Geometry check sheet. Reference: the model listing, model coordinates, mm. Give positions to 0.01 mm unless a question says otherwise; leave off trailing zeros. Order: outer loops, then holes, each group sorted by start corner. A loop starts at its lowest first (then second) coordinate and runs counter-clockwise, first axis right, second up. Notation, with made-up numbers: M -12,25.25 L 44,25.25 A23 cw 44,46.25 Z; hole C 5.25,52.5 d9. An arc over 180 degrees is marked long. One line per question, with ' | ' between items. Start each with the question number.
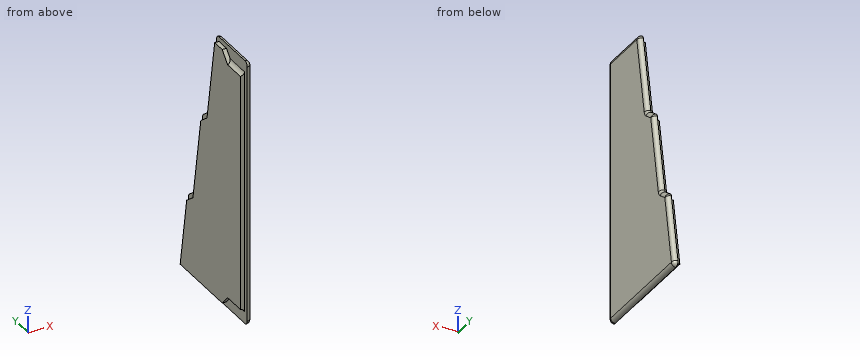
from build123d import *

# Parameters (mm, degrees)
BOSS_EXTRUDE1_DEPTH  = 3
FILLET1_R            = 3
BOSS_EXTRUDE2_DEPTH  = 3
CUT_EXTRUDE1_START   = -16.870694295
CUT_EXTRUDE1_DEPTH   = 17.870694295
CUT_EXTRUDE1_START_2 = 6.082684495
CUT_EXTRUDE1_2_DEPTH = 3.553569774
CUT_EXTRUDE1_START_3 = -94.677172909
CUT_EXTRUDE1_3_DEPTH = 3.677172909
CUT_EXTRUDE2_REACH   = 418.489


with BuildPart() as part:
    # Sketch1 → Boss-Extrude1 (new body)
    with BuildSketch(Plane.ZY.offset(376.423184311)):
        with BuildLine():
            Line((-33.382889261, -4.0880098), (-33.382889261, -11.0880098))
            ThreePointArc((-33.382889261, -11.0880098), (-32.504209605, -13.209330144), (-30.382889261, -14.0880098))
            Line((-30.382889261, -14.0880098), (147.429996243, -14.0880098))
            ThreePointArc((147.429996243, -14.0880098), (149.551316587, -13.209330144), (150.429996243, -11.0880098))
            Line((150.429996243, -11.0880098), (150.429996243, -4.0880098))
            Line((150.429996243, -4.0880098), (150.429996243, 23.394691306))
            ThreePointArc((150.429996243, 23.394691306), (149.728129572, 25.323054136), (147.950940776, 26.349114566))
            Line((147.950940776, 26.349114566), (92.565293245, 36.115098569))
            ThreePointArc((92.565293245, 36.115098569), (91.474338953, 36.539347491), (90.628781645, 37.348792519))
            Line((90.628781645, 37.348792519), (86.318516116, 43.504489644))
            ThreePointArc((86.318516116, 43.504489644), (85.472958808, 44.313934672), (84.382004516, 44.738183594))
            Line((84.382004516, 44.738183594), (27.741063701, 54.725509672))
            ThreePointArc((27.741063701, 54.725509672), (26.650109409, 55.149758594), (25.804552101, 55.959203622))
            Line((25.804552101, 55.959203622), (21.494286572, 62.114900747))
            ThreePointArc((21.494286572, 62.114900747), (20.648729264, 62.924345775), (19.557774972, 63.348594697))
            Line((19.557774972, 63.348594697), (-29.861944728, 72.062624659))
            ThreePointArc((-29.861944728, 72.062624659), (-32.31125209, 71.406334729), (-33.382889261, 69.1082014))
            Line((-33.382889261, 69.1082014), (-33.382889261, -4.0880098))
        make_face()
    extrude(amount=BOSS_EXTRUDE1_DEPTH)

    # Fillet1
    fillet1_edges = [part.edges().sort_by_distance(p)[0] for p in [
        (-379.423184311, 67.705609678, -5.152084878),
        (-379.423184311, 62.924345775, 20.648729264),
        (-379.423184311, 59.037052184, 23.649419336),
        (-379.423184311, 55.149758594, 26.650109409),
        (-379.423184311, 49.731846633, 56.061534109),
        (-379.423184311, 44.313934672, 85.472958808),
        (-379.423184311, 40.426641081, 88.473648881),
        (-379.423184311, 36.539347491, 91.474338953),
        (-379.423184311, 31.232106567, 120.258117011),
        (-379.423184311, 25.323054136, 149.728129572),
        (-379.423184311, 6.153340753, 150.429996243),
        (-379.423184311, -13.209330144, 149.551316587),
        (-379.423184311, -14.0880098, 58.523553491),
        (-379.423184311, -13.209330144, -32.504209605),
        (-379.423184311, 29.0100958, -33.382889261),
        (-379.423184311, 71.406334729, -32.31125209),
    ]]
    fillet(fillet1_edges, radius=FILLET1_R - 0.0001)  # a hair under: the kernel refuses the full size

    # Sketch2 → Boss-Extrude2 (add)
    with BuildSketch(Plane(origin=(-376.423184311, 0, 0), x_dir=(0, 0, -1), z_dir=(1, 0, 0))):
        Polygon((-147.129996243, 23.142961417), (-147.129996243, 13.236254269), (-143.529996243, 9.636254269), (-143.529996243, -4.0880098), (-143.529996243, -10.7880098), (26.482889261, -10.7880098), (26.482889261, -4.0880098), (26.482889261, 9.636254269), (30.082889261, 13.236254269), (30.082889261, 68.750675322), (-18.862359767, 60.120307341), (-24.598124131, 51.928786898), (-83.686589311, 41.509896238), (-89.422353675, 33.318375795), align=None)
    extrude(amount=BOSS_EXTRUDE2_DEPTH)

    # Cut-Extrude1: read off the stored shape, not the designer's step
    # Cut-Extrude1 outline → Cut-Extrude1 (cut)
    with BuildSketch(Plane.XZ.offset(10.7880098).offset(CUT_EXTRUDE1_START)):
        with BuildLine():
            Line((-376.423184311, 143.529996243), (-376.423184311, 142.329996243))
            ThreePointArc((-376.423184311, 142.329996243), (-375.230428102, 140.761580148), (-373.423184311, 139.97642647))
            Line((-373.423184311, 139.97642647), (-373.423184311, 143.529996243))
            Line((-373.423184311, 143.529996243), (-376.423184311, 143.529996243))
        make_face()
    extrude(amount=CUT_EXTRUDE1_DEPTH, mode=Mode.SUBTRACT)

    # Cut-Extrude1 2 outline → Cut-Extrude1 2 (cut)
    with BuildSketch(Plane(origin=(0, 0, 0), x_dir=(1, 0, 0), z_dir=(0, 1, 0)).offset(CUT_EXTRUDE1_START_2)):
        with BuildLine():
            ThreePointArc((-373.423184311, -139.97642647), (-375.230428102, -140.761580148), (-376.423184311, -142.329996243))
            Line((-376.423184311, -142.329996243), (-376.423184311, -143.529996243))
            Line((-376.423184311, -143.529996243), (-373.423184311, -143.529996243))
            Line((-373.423184311, -143.529996243), (-373.423184311, -139.97642647))
        make_face()
    extrude(amount=CUT_EXTRUDE1_2_DEPTH, mode=Mode.SUBTRACT)

    # Cut-Extrude1 3 outline → Cut-Extrude1 3 (add)
    with BuildSketch(Plane(origin=(0, 0, 0), x_dir=(1, 0, 0), z_dir=(0, 0.707106781186553, -0.707106781186542)).offset(CUT_EXTRUDE1_START_3)):
        with BuildLine():
            Line((-376.423184311, -106.607838111), (-376.423184311, -113.39606321))
            Line((-376.423184311, -113.39606321), (-373.423184311, -113.39606321))
            Line((-373.423184311, -113.39606321), (-373.423184311, -103.279387817))
            add(Edge.make_bspline(
                [(-373.423184311, -103.279387817), (-375.582623677, -103.754880716), (-376.423184311, -106.607838111)],
                knots=[0.154459598, 0.154459598, 0.154459598, 1.176005207, 1.176005207, 1.176005207], degree=2, weights=[1, 0.872366982, 1]))
        make_face()
    extrude(amount=CUT_EXTRUDE1_3_DEPTH)

    # Cut-Extrude2: up to this plane
    cut_extrude2_end = Plane(origin=(-373.423184311, -8.423317496, -8.423317496), z_dir=(0, 0.7071067811865445, 0.7071067811865507))
    # Sketch3<3> → Cut-Extrude2 (cut, up to the surface)
    with BuildSketch(Plane.XZ.offset(10.7880098), mode=Mode.PRIVATE) as cut_extrude2_sk1:
        with BuildLine():
            Line((-373.423184311, -26.482889261), (-373.423184311, -23.233241391))
            ThreePointArc((-373.423184311, -23.233241391), (-375.473428882, -24.346456682), (-376.410662534, -26.482889261))
            Line((-376.410662534, -26.482889261), (-373.423184311, -26.482889261))
        make_face()
    cut_extrude2_tool1 = split(extrude(cut_extrude2_sk1.sketch, amount=-CUT_EXTRUDE2_REACH, mode=Mode.PRIVATE), bisect_by=cut_extrude2_end, keep=Keep.BOTH, mode=Mode.PRIVATE)
    add(cut_extrude2_tool1.solids().sort_by_distance((-374.649681, -10.78801, -25.160842))[0], mode=Mode.SUBTRACT)
    # Sketch3<3> → Cut-Extrude2 (cut, up to the surface)
    with BuildSketch(Plane.XZ.offset(10.7880098), mode=Mode.PRIVATE) as cut_extrude2_sk2:
        with BuildLine():
            ThreePointArc((-373.473184311, -22.937437402), (-375.250304231, -23.730170981), (-376.423184311, -25.282889261))
            Line((-376.423184311, -25.282889261), (-376.423184311, -26.482889261))
            Line((-376.423184311, -26.482889261), (-376.410662534, -26.482889261))
            ThreePointArc((-376.410662534, -26.482889261), (-375.473428882, -24.346456682), (-373.423184311, -23.233241391))
            Line((-373.423184311, -23.233241391), (-373.423184311, -22.929319487))
            ThreePointArc((-373.423184311, -22.929319487), (-373.448197491, -22.933297266), (-373.473184311, -22.937437402))
        make_face()
    cut_extrude2_tool2 = split(extrude(cut_extrude2_sk2.sketch, amount=-CUT_EXTRUDE2_REACH, mode=Mode.PRIVATE), bisect_by=cut_extrude2_end, keep=Keep.BOTH, mode=Mode.PRIVATE)
    add(cut_extrude2_tool2.solids().sort_by_distance((-373.46969, -10.78801, -23.08128))[0], mode=Mode.SUBTRACT)


with BuildPart() as body_2:
    # Mirror1: mirrored copy
    add(part.part.mirror(Plane(origin=(-373.423184311, 0, 0), x_dir=(0, 0, 1), z_dir=(1, 0, 0))))


solid = body_2.part
Item 1: Depth check by flat-ended pin: pin 1 (2 mm diameter, centred on x = -368, z = 67, fed in from +Y); pin 2 (2.5 mm diameter, centred on x = -372, z = 20.5, fed in from -Y); pin 3 (0.9 mm diameter, centred on x = -372, y = 16, fed in from +Z). Enter the tip coordinate at first touch or a pass-through.
Item 2: Cross-section at A-A, the plane x = -371.5. Record the cut outline in (y, z), plus the area to 3 significant figures.
Item 3: Material ranges on line 1 along Y through (x, z) = (-371, 25.5); line 2 along Y through (x, z) = (-372.25, 129); line 3 along X through (y, z) = (63, 8), recorded low to high.
Outcome:
1) pin 1: stops at y = 47.47 | pin 2: stops at y = -10.79 | pin 3: stops at z = 147.13
2) outline: M -10.79,-23.81 L 6.96,-23.81 L 13.24,-30.08 L 68.75,-30.08 L 60.12,18.86 L 51.93,24.6 L 41.51,83.69 L 33.32,89.42 L 23.14,147.13 L 13.24,147.13 L 6.96,140.86 L -10.79,140.86 Z | area: 9,730 mm²
3) line 1: y = -10.79 to 51.77 | line 2: y = -10.79 to 26.34 | line 3: x = -370.42 to -367.49
